```python
from build123d import *

# Parameters (mm, degrees)
F0_R     = 9.525
F0_R_2   = 58
F1_DEPTH = 6.35


# Not quite as in the source:
# - a feature names something its author has since deleted; it is built from what else it names


with BuildPart() as f1:
    # F0 (on Front) → F1 (new body, symmetric)
    with BuildSketch(Plane.XZ):
        with BuildLine():
            Line((14.4609105581, 197.3757855088), (-239.8028006456, -342.2453456239))
            ThreePointArc((-239.8028006456, -342.2453456239), (-225.7250673292, -396.6962310463), (-169.6171250668, -392.8257900262))
            Line((-169.6171250668, -392.8257900262), (59.9480115155, -173.6686590313))
            ThreePointArc((59.9480115155, -173.6686590313), (91.8054714835, -153.1745344831), (129, -146))
            Line((129, -146), (664, -146))
            Line((664, -146), (764, -66))
            Line((764, -66), (764, -46))
            Line((764, -46), (149, -46))
            ThreePointArc((149, -46), (131.3223304703, -38.6776695297), (124, -21))
            Line((124, -21), (124, 390))
            Line((124, 390), (104, 390))
            Line((104, 390), (24, 290))
            Line((24, 290), (24, 240))
            ThreePointArc((24, 240), (21.5860929022, 218.1607126469), (14.4609105581, 197.3757855088))
        make_face()
        with Locations((-200, -361)):
            Circle(F0_R, mode=Mode.SUBTRACT)
        Circle(F0_R_2, mode=Mode.SUBTRACT)
    extrude(amount=F1_DEPTH, both=True)


solid = f1.part
```
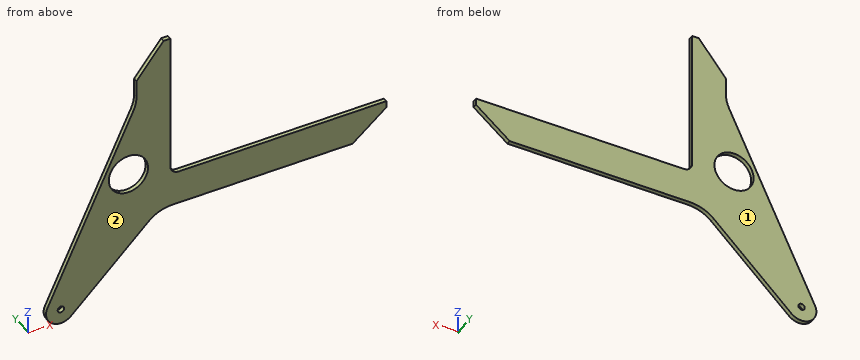
Geometry check sheet. Reference: the model listing, model coordinates, mm. Face numbers are marked on the shaded views. Give positions to 0.01 mm unless a question says otherwise; leave off trailing zeros. Loops run counter-clockwise (first coordinate to the right, second up) from the corner with the lowest first, then second, coordinate; pieces in that order, holes last. Notation, with made-up numbers: M -20,-27 L 30,-27 A12 ccw 30,-4 Z; hole C -5.75,56 d8. An arc over 180 degrees is marked long. Write item = value, one per line. Start each with the question number.
1. Section check C-C, the plane x = 0. Enter the section's corners in (y, z), plus the area to 3 significant figures.
2. Go/stop test with flat-tipped pins: P1, Ø17, axis at x = -200, z = -361, coming from the -Y side; P2, Ø1, axis at x = 6, y = 1.5, coming from the -Z side; P3, Ø5, axis at y = 3.5, z = -97.5, coming from the +X side; P4, Ø5, axis at x = 60, y = 4.5, coming from the -Z side. Record where each tip stops, or that it passes through.
3. Section check D-D, the plane x = 677. Enter the section's corners in (y, z).
4. Draft check along Y on the marked faces 1 and 2. Enter one of: +Y half, -Y half, draft (parallel to the pull), parting line (faces both ways), or undercut.
5. Section check B-B, the plane z = 13. Enter the section's corners in (x, y).
6. Thickness scan on probe 1 along Z at (x, y) = (305, -1.5); probe 2 along Z at (x, y) = (-200, -1.5) (3 decimals); probe 3 along X at (y, z) = (-5.25, -52). Record the ranges inside material, lowest first.
7. Section check A-A, the plane y = 1.25. Enter the section's corners in (x, z) (3 decimals).
Values follow:
q1.outline = M -6.35,-230.9 L 6.35,-230.9 L 6.35,-58 L -6.35,-58 Z; M -6.35,58 L 6.35,58 L 6.35,166.69 L -6.35,166.69 Z
q1.area = 3,580 mm^2
q2.P1 = through
q2.P2 = -225.65
q2.P3 = 727.75
q2.P4 = -176.01
q3.outline = M -6.35,-135.6 L 6.35,-135.6 L 6.35,-46 L -6.35,-46 Z
q4.face_1 = +Y half
q4.face_2 = -Y half
q5.outline = M -72.41,-6.35 L -56.52,-6.35 L -56.52,6.35 L -72.41,6.35 Z; M 56.52,-6.35 L 124,-6.35 L 124,6.35 L 56.52,6.35 Z
q6.probe_1 = -146 to -46
q6.probe_2 = -405 to -370.525, -351.475 to -257.772
q6.probe_3 = -103.04 to -25.69, 25.69 to 764
q7.outline = M -239.803,-342.245 A44 ccw -169.617,-392.826 L 59.948,-173.669 A100 cw 129,-146 L 664,-146 L 764,-66 L 764,-46 L 149,-46 A25 cw 124,-21 L 124,390 L 104,390 L 24,290 L 24,240 A100 cw 14.461,197.376 Z; hole C -200,-361 d19.05; hole C 0,0 d116
